from build123d import *

# Parameters (mm, degrees)
SKETCH1_W               = 220
SKETCH1_H               = 145
SKETCH1_W_2             = 42.5
SKETCH1_H_2             = 52.5
BOSS_EXTRUDE1_DEPTH     = 3
SKETCH2_W               = 220
SKETCH2_H               = 145
BOSS_EXTRUDE2_DEPTH     = 37
SKETCH3_W               = 27.3375
SKETCH3_H               = 19.05
CUT_EXTRUDE1_DEPTH      = 3
SKETCH3_6_W             = 53.975
SKETCH3_6_H             = 31.75
CUT_EXTRUDE2_DEPTH      = 8.5
CUT_EXTRUDE3_DEPTH      = 267.505159425
CUT_EXTRUDE3_DEPTH_BACK = 267.505159425
CUT_EXTRUDE4_DEPTH      = 267.071418984
CUT_EXTRUDE4_DEPTH_BACK = 267.071418984


with BuildPart() as part:
    # Sketch1 → Boss-Extrude1 (new body)
    with BuildSketch(Plane(origin=(0, 0, 0), x_dir=(1, 0, 0), z_dir=(0, 1, 0))):
        with Locations((110, 72.5)):
            Rectangle(SKETCH1_W, SKETCH1_H)
        Polygon((10, 82.5), (52.5, 82.5), (52.5, 135), (31.25, 135), (10, 108.75), align=None, mode=Mode.SUBTRACT)
        with Locations((83.75, 108.75)):
            Rectangle(SKETCH1_W_2, SKETCH1_H_2, mode=Mode.SUBTRACT)
        with Locations((83.75, 36.25)):
            Rectangle(SKETCH1_W_2, SKETCH1_H_2, mode=Mode.SUBTRACT)
        Polygon((10, 36.25), (31.25, 10), (52.5, 10), (52.5, 62.5), (10, 62.5), align=None, mode=Mode.SUBTRACT)
        Polygon((210, 62.5), (210, 36.25), (188.75, 10), (167.5, 10), (167.5, 62.5), align=None, mode=Mode.SUBTRACT)
        with Locations((136.25, 36.25)):
            Rectangle(SKETCH1_W_2, SKETCH1_H_2, mode=Mode.SUBTRACT)
        with Locations((136.25, 108.75)):
            Rectangle(SKETCH1_W_2, SKETCH1_H_2, mode=Mode.SUBTRACT)
        Polygon((210, 108.75), (188.75, 135), (167.5, 135), (167.5, 82.5), (210, 82.5), align=None, mode=Mode.SUBTRACT)
    extrude(amount=BOSS_EXTRUDE1_DEPTH)

    # Sketch2 → Boss-Extrude2 (add)
    with BuildSketch(Plane(origin=(0, 3, 0), x_dir=(1, 0, 0), z_dir=(0, 1, 0))):
        with Locations((110, 72.5)):
            Rectangle(SKETCH2_W, SKETCH2_H)
        with BuildLine():
            Line((3, 123.3), (3, 21.7))
            ThreePointArc((3, 21.7), (9.01040764, 19.21040764), (11.5, 13.2))
            Line((11.5, 13.2), (11.5, 3))
            Line((11.5, 3), (208.5, 3))
            Line((208.5, 3), (208.5, 13.2))
            ThreePointArc((208.5, 13.2), (210.98959236, 19.21040764), (217, 21.7))
            Line((217, 21.7), (217, 123.3))
            ThreePointArc((217, 123.3), (210.98959236, 125.78959236), (208.5, 131.8))
            Line((208.5, 131.8), (208.5, 142))
            Line((208.5, 142), (11.5, 142))
            Line((11.5, 142), (11.5, 131.8))
            ThreePointArc((11.5, 131.8), (9.01040764, 125.78959236), (3, 123.3))
        make_face(mode=Mode.SUBTRACT)
    extrude(amount=BOSS_EXTRUDE2_DEPTH)

    # Sketch3 → Cut-Extrude1 (cut)
    with BuildSketch(Plane.ZY.offset(-3)):
        with Locations((-35.36875, 18.478125)):
            Rectangle(SKETCH3_W, SKETCH3_H)
    extrude(amount=CUT_EXTRUDE1_DEPTH, mode=Mode.SUBTRACT)

    # Sketch3<6> → Cut-Extrude2 (cut)
    with BuildSketch(Plane.ZY.offset(-3)):
        with Locations((-29.9875, 18.875)):
            Rectangle(SKETCH3_6_W, SKETCH3_6_H)
    extrude(amount=-CUT_EXTRUDE2_DEPTH, mode=Mode.SUBTRACT)

    # Sketch7 → Cut-Extrude3 (cut, two sides)
    with BuildSketch(Plane.XY) as cut_extrude3_sk:
        Polygon((110, 40), (110, 34.333333333), (105, 29.333333333), (110, 24.333333333), (110, 18.666666667), (115, 13.666666667), (110, 8.666666667), (110, 3), (220, 3), (220, 40), align=None)
    extrude(amount=CUT_EXTRUDE3_DEPTH, mode=Mode.SUBTRACT)
    extrude(cut_extrude3_sk.sketch, amount=-CUT_EXTRUDE3_DEPTH_BACK, mode=Mode.SUBTRACT)

    # Sketch8 → Cut-Extrude4 (cut, two sides)
    with BuildSketch(Plane(origin=(0, 3, 0), x_dir=(1, 0, 0), z_dir=(0, 1, 0))) as cut_extrude4_sk:
        Polygon((110, 145), (220, 145), (220, 0), (110, 0), (110, 17.095598855), (106.464466094, 20.631132761), (110, 24.166666667), (110, 41.262265521), (106.464466094, 44.797799427), (110, 48.333333333), (110, 65.428932188), (106.464466094, 68.964466094), (113.535533906, 76.035533906), (110, 79.571067812), (110, 96.666666667), (113.535533906, 100.202200573), (110, 103.737734479), (110, 120.833333333), (113.535533906, 124.368867239), (110, 127.904401145), align=None)
    extrude(amount=CUT_EXTRUDE4_DEPTH, mode=Mode.SUBTRACT)
    extrude(cut_extrude4_sk.sketch, amount=-CUT_EXTRUDE4_DEPTH_BACK, mode=Mode.SUBTRACT)


solid = part.part
Design review of the part built by this model. Coordinates are the model's own, in mm. A direction names the side the tool comes from. Round coordinates to 2 decimals unless told otherwise and drop trailing zeros. Loops run counter-clockwise (first coordinate to the right, second up) from the corner with the lowest first, then second, coordinate; pieces in that order, holes last. Notation, with made-up numbers: (-8.75, 25.5) -> (0.25, 25.5) arc R19 ccw to (0.25, 46.5) -> close; hole circle Ø8 at (49.25, -38.5). An arc over 180 degrees is marked (long way). Use one line per item in the form item = value. Start each with the question number.
Q1. Machinability: for faces 1 (the face through (2, 18, -49.037)), 2 (the face through (9.08, 21.24, -125.86)), 3 (the face through (110, 2, -112)), 4 (the face through (62.5, 1, -36)), 5 (the face through (110, 10.4, -2.8)), which of the approach directions +Z, -Z, +X, -X, +Y, -Y give a long, thin tool a straight path to every point of the face, cutting with its end or side? Answer none if there is none.
Q2. We need section A-A on y = 10.5. Give the boundary of the cut face in (x, z), then the cut area to 3 significant figures.
Q3. Draft analysis for pull direction Z (two halves, no side actions). For faces 6 (the face through (110, 10, -143)), 7 (the face through (108.207, 1.521, -46.541)), 8 (the face through (54, 20, -145)), state which applies: +Z half, -Z half, draft (parallel to the pull), parting line (faces both ways), or undercut.
Q4. Wall thickness on line 1 along Z through (x, y) = (42.5, 26.5); line 2 along X through (y, z) = (27.5, -85.5): over which ranges is each line inside the solid? List them lowest first. Write a range as [from, to].
Q5. We need section C-C on z = -56.5. Give the boundary of the cut face in (x, y), then the cut area to 3 significant figures.
Q6. We need section B-B on x = 84. Give the boundary of the cut face in (y, z), then the cut area to 3 significant figures.
Q7. We need section D-D on x = 13.5. Give the boundary of the cut face in (y, z), then the cut area to 3 significant figures.
Q8. For pin 1 Ø4 at (y, z) = (37, -6.5) entering from +X; pin 2 Ø0.9 at (y, z) = (2, -54) entering from +X, all flat-tipped, find the tip position at first contact; note any pin that passes through.
Calculated:
q1.face_1 = +X, -X
q1.face_2 = +X, +Y
q1.face_3 = +X, +Y, -Y
q1.face_4 = +Y, -Y
q1.face_5 = +Z, +X, +Y, -Y
q2.outline = (0, -145) -> (110, -145) -> (110, -142) -> (11.5, -142) -> (11.5, -131.8) arc R8.5 ccw to (3, -123.3) -> (3, -49.04) -> (0, -49.04) -> close; (0, -21.7) -> (3, -21.7) -> (3, -3) -> (110, -3) -> (110, 0) -> (0, 0) -> close
q2.area = 1,140 mm²
q3.face_6 = draft
q3.face_7 = undercut
q3.face_8 = -Z half
q4.line_1 = [-145, -142], [-3, 0]
q4.line_2 = [0, 3]
q5.outline = (0, 0) -> (10, 0) -> (10, 3) -> (3, 3) -> (3, 40) -> (0, 40) -> close; (52.5, 0) -> (62.5, 0) -> (62.5, 3) -> (52.5, 3) -> close; (105, 0) -> (110, 0) -> (110, 3) -> (105, 3) -> close
q5.area = 186 mm²
q6.outline = (0, -145) -> (40, -145) -> (40, -142) -> (3, -142) -> (3, -135) -> (0, -135) -> close; (0, -82.5) -> (3, -82.5) -> (3, -62.5) -> (0, -62.5) -> close; (0, -10) -> (3, -10) -> (3, -3) -> (40, -3) -> (40, 0) -> (0, 0) -> close
q6.area = 342 mm²
q7.outline = (0, -145) -> (40, -145) -> (40, -142) -> (3, -142) -> (3, -113.07) -> (0, -113.07) -> close; (0, -82.5) -> (3, -82.5) -> (3, -62.5) -> (0, -62.5) -> close; (0, -31.93) -> (3, -31.93) -> (3, -3) -> (40, -3) -> (40, 0) -> (0, 0) -> close
q7.area = 474 mm²
q8.pin_1 = 11.5
q8.pin_2 = 110
